```python
from build123d import *

# Parameters (mm, degrees)
SKETCH1_W                       = 25.4
SKETCH1_H                       = 76.2
SKETCH1_W_2                     = 19.05
SKETCH1_H_2                     = 69.85
BOSS_EXTRUDE1_DEPTH             = 279.4
SKETCH3_R                       = 1.7272
CUT_EXTRUDE2_DEPTH              = 6.35
F_1_4_0_25_DIAMETER_HOLE1_D     = 6.35
F_1_4_0_25_DIAMETER_HOLE1_DEPTH = 25.4
F_1_4_0_25_DIAMETER_HOLE1_TIP   = 1.907732465
F_1_4_0_25_DIAMETER_HOLE2_D     = 6.35
SKETCH2_R                       = 1.7272
CUT_EXTRUDE4_DEPTH              = 6.35


with BuildPart() as part:
    # Sketch1 → Boss-Extrude1 (new, symmetric)
    with BuildSketch(Plane.XY):
        Rectangle(SKETCH1_W, SKETCH1_H)
        Rectangle(SKETCH1_W_2, SKETCH1_H_2, mode=Mode.SUBTRACT)
    extrude(amount=BOSS_EXTRUDE1_DEPTH, both=True)

    # Sketch3 → Cut-Extrude2 (cut)
    with BuildSketch(Plane.XZ.offset(38.1)):
        with Locations(Location((0, 254, 0), (0, 0, 270))):
            Circle(SKETCH3_R)
        with Locations(Location((0, 203.2, 0), (0, 0, 270))):
            Circle(SKETCH3_R)
        with Locations(Location((0, 152.4, 0), (0, 0, 270))):
            Circle(SKETCH3_R)
        with Locations(Location((0, 101.6, 0), (0, 0, 270))):
            Circle(SKETCH3_R)
        with Locations(Location((0, 50.8, 0), (0, 0, 270))):
            Circle(SKETCH3_R)
        with Locations(Location((0, 0, 0), (0, 0, 270))):
            Circle(SKETCH3_R)
        with Locations(Location((0, -50.8, 0), (0, 0, 270))):
            Circle(SKETCH3_R)
        with Locations(Location((0, -101.6, 0), (0, 0, 270))):
            Circle(SKETCH3_R)
        with Locations(Location((0, -152.4, 0), (0, 0, 270))):
            Circle(SKETCH3_R)
        with Locations(Location((0, -203.2, 0), (0, 0, 270))):
            Circle(SKETCH3_R)
        with Locations(Location((0, -254, 0), (0, 0, 270))):
            Circle(SKETCH3_R)
    extrude(amount=-CUT_EXTRUDE2_DEPTH, mode=Mode.SUBTRACT)

    # 1/4 (0.25) Diameter Hole1
    with Locations(Plane.ZY.offset(12.7)):
        with Locations((-60.325, -28.575), (60.325, -28.575), (-60.325, -9.525), (60.325, -9.525)):
            Hole(F_1_4_0_25_DIAMETER_HOLE1_D / 2, depth=F_1_4_0_25_DIAMETER_HOLE1_DEPTH)
            with Locations((0, 0, -(F_1_4_0_25_DIAMETER_HOLE1_DEPTH + F_1_4_0_25_DIAMETER_HOLE1_TIP / 2))):  # 118° drill point
                Cone(0, F_1_4_0_25_DIAMETER_HOLE1_D / 2, F_1_4_0_25_DIAMETER_HOLE1_TIP, mode=Mode.SUBTRACT)

    # 1/4 (0.25) Diameter Hole2 (through all)
    with Locations(Plane(origin=(0, 38.1, 0), x_dir=(1, 0, 0), z_dir=(0, 1, 0))):
        with Locations((0, -38.1), (0, 38.1)):
            Hole(F_1_4_0_25_DIAMETER_HOLE2_D / 2)

    # Sketch2 → Cut-Extrude4 (cut)
    with BuildSketch(Plane(origin=(0, 38.1, 0), x_dir=(1, 0, 0), z_dir=(0, 1, 0))):
        with Locations(Location((0, 266.7, 0), (0, 0, 270))):
            Circle(SKETCH2_R)
        with Locations(Location((0, 241.3, 0), (0, 0, 270))):
            Circle(SKETCH2_R)
        with Locations(Location((0, 215.9, 0), (0, 0, 270))):
            Circle(SKETCH2_R)
        with Locations(Location((0, 190.5, 0), (0, 0, 270))):
            Circle(SKETCH2_R)
        with Locations(Location((0, 165.1, 0), (0, 0, 270))):
            Circle(SKETCH2_R)
    cut_extrude4 = extrude(amount=-CUT_EXTRUDE4_DEPTH, mode=Mode.SUBTRACT)

    # Mirror1: Cut-Extrude4 across plane
    add(cut_extrude4.mirror(Plane.XY), mode=Mode.SUBTRACT)


solid = part.part
```
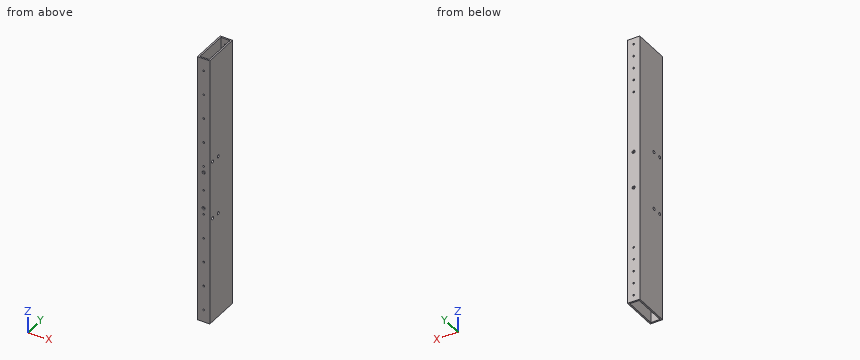
For this review, take the finished solid that the model builds, in its own axes (mm). Give positions to 0.01 mm unless a question says otherwise; leave off trailing zeros. Write each loop counter-clockwise with the first axis right and the second up, starting at its lowest first coordinate (ties: lowest second). Pieces come first, ordered by that corner, then holes.
Item 1: Wall thickness on probe 1 along X at (y, z) = (-28, 194) (3 decimals); probe 2 along Y at (x, z) = (-5, -79.5) (3 decimals); probe 3 along X at (y, z) = (36.4, 215.9): over which ranges is each line inside the solid? List them lowest first.
Item 2: Take a section at A-A (z = 227). Give the boundary of the cut face in (x, y) (3 decimals), and give its area (3 significant figures).
Item 3: Insertion check: P1, Ø2, axis at x = 0, z = 266.7, coming from the +Y side (3 decimals); P2, Ø3, axis at x = -6.5, y = -29, coming from the +Z side; P3, Ø3, axis at x = 0, z = -203.2, coming from the -Y side (3 decimals). Each pin has a flat end and moves straight along its axis. Give the tip position at first contact, or say it passes through.
Established:
1. probe 1: x = -12.7 to -9.525, 9.525 to 12.7
1. probe 2: y = -38.1 to -34.925, 34.925 to 38.1
1. probe 3: x = -12.7 to -1.73, 1.73 to 12.7
2. outline: (-12.7, -38.1) - (12.7, -38.1) - (12.7, 38.1) - (-12.7, 38.1) - close; hole (-9.525, -34.925) - (9.525, -34.925) - (9.525, 34.925) - (-9.525, 34.925) - close
2. area: 605 mm2
3. P1: stops at y = -34.925
3. P2: passes through
3. P3: stops at y = 34.925
